from build123d import *

# Parameters (mm, degrees)
BOSS_EXTRUDE1_DEPTH = 38.1
CUT_EXTRUDE1_DEPTH  = 2.54
CUT_EXTRUDE2_DEPTH  = 34.29
BOSS_EXTRUDE2_DEPTH = 25.4
SHELL1_START        = -12.546191045
SHELL1_DEPTH        = 24.13
SHELL1_2_DEPTH      = 22.86


# Read off the part's stored shape, not the designer's step: Shell1
with BuildPart() as part:
    # Sketch1 → Boss-Extrude1 (new body)
    with BuildSketch(Plane(origin=(0, 0, 0), x_dir=(1, 0, 0), z_dir=(0, 1, 0))):
        Polygon((12.853808955, 0.174987325), (12.853808955, 37.417012675), (82.296, 25.146), (82.296, 12.446), align=None)
    extrude(amount=BOSS_EXTRUDE1_DEPTH)

    # Sketch3 → Cut-Extrude1 (cut)
    with BuildSketch(Plane(origin=(0, 35.56, 0), x_dir=(1, 0, 0), z_dir=(0, 1, 0))):
        Polygon((79.756, 14.576512841), (79.756, 23.015487159), (15.393808955, 34.388821586), (15.393808955, 3.203178414), align=None)
    extrude(amount=CUT_EXTRUDE1_DEPTH, mode=Mode.SUBTRACT)

    # Sketch6 → Cut-Extrude2 (cut)
    with BuildSketch(Plane(origin=(0, 35.56, 0), x_dir=(1, 0, 0), z_dir=(0, 1, 0))):
        Polygon((81.026, 13.511256421), (81.026, 24.080743579), (14.123808955, 35.90291713), (14.123808955, 1.68908287), align=None)
    extrude(amount=-CUT_EXTRUDE2_DEPTH, mode=Mode.SUBTRACT)

    # Sketch8 → Boss-Extrude2 (add)
    with BuildSketch(Plane.ZY.offset(-12.853808955)):
        Polygon((-31.26502256, 38.1), (-31.26502256, 0), (-18.796, 2.1986251), (-6.32697744, 0), (-6.32697744, 38.1), (-18.796, 40.2986251), align=None)
    extrude(amount=BOSS_EXTRUDE2_DEPTH)

    # Shell1 outline → Shell1 (cut)
    with BuildSketch(Plane.YZ.offset(SHELL1_START)):
        Polygon((35.56, -28.72502256), (35.56, -8.86697744), (3.027054125, -8.86697744), (4.777808695, -18.796), (3.027054125, -28.72502256), align=None)
    extrude(amount=SHELL1_DEPTH, mode=Mode.SUBTRACT)

    # Shell1 2 outline → Shell1 2 (cut)
    with BuildSketch(Plane.YZ.offset(SHELL1_START)):
        Polygon((35.968686937, -8.86697744), (35.56, -8.86697744), (35.56, -28.72502256), (35.968686937, -28.72502256), (37.719441506, -18.796), align=None)
    extrude(amount=SHELL1_2_DEPTH, mode=Mode.SUBTRACT)


solid = part.part
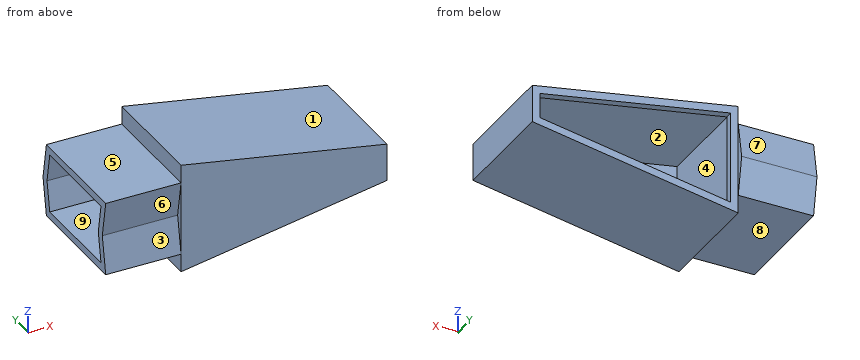
Source: CAD feature listing. Evaluate the final solid. Frame: model axes, mm. Face numbers are marked on the shaded views. A direction names the side the tool comes from. Round coordinates to 2 decimals unless told otherwise and drop trailing zeros. Loops run counter-clockwise (first coordinate to the right, second up) from the corner with the lowest first, then second, coordinate; pieces in that order, holes last. Notation, with made-up numbers: (-22, 29) -> (3, 29) arc R22 ccw to (3, 53) -> close; hole circle Ø5 at (53.5, -28.5). An arc over 180 degrees is marked (long way). Answer as a JSON object with one key per item and string values. Group by question number.
Q1. Section query D-D (x = 55.5). Output: boundary loops of the cut face in (y, z), plus the area to 3 significant figures.
Q2. Mould query, pull axis X, two halves, no side actions, for the marked faces 1, 2, 3 and 4. Classes: pulls with the +X half, pulls with the -X half, needs draft (parallel to the pull), parting line crosses it, or undercut.
Q3. Contact query for flat-ended pins moving along their axis: P1, Ø8, axis at x = 0.5, z = -29, coming from the -Y side; P2, Ø12, axis at x = 25.5, y = 16.5, coming from the -Z side; P3, Ø2.5, axis at y = 39.5, z = -19.5, coming from the +X side. Output: stop coordinate, or through.
Q4. Section query A-A (y = 11). Output: boundary loops of the cut face in (x, z), plus the area to 3 significant figures.
Q5. Access query for the marked faces 5, 6, 7, 8 and 9. Directions: +Z, -Z, +X, -X, +Y, -Y. A direction counts if a zero-diameter tool reaches every point of the face in a straight line with its end or side. Return the directions, or none.
Q6. Section query B-B (x = 71.5). Output: boundary loops of the cut face in (y, z), plus the area to 3 significant figures.
Q7. Ray query, line 1 (Z direction, x = -1.5, y = 10); line 2 (X direction, y = 27, z = -22); line 3 (Y direction, x = 33, z = -17). Return the intervals inside material, ascending. Write a range as from..to.
Q8. Section query C-C (z = -21). Output: boundary loops of the cut face in (x, y), plus the area to 3 significant figures.
Completed:
{
 "1": {"outline": "(0, -29.88) -> (38.1, -29.88) -> (38.1, -27.3) -> (35.56, -27.3) -> (35.56, -28.59) -> (1.27, -28.59) -> (1.27, -9) -> (35.56, -9) -> (35.56, -10.29) -> (38.1, -10.29) -> (38.1, -7.71) -> (0, -7.71) -> close", "area": "130 mm²"},
 "2": {"face 1": "pulls with the +X half", "face 2": "undercut", "face 3": "needs draft", "face 4": "undercut"},
 "3": {"P1": "y = 0", "P2": "z = -36.24", "P3": "x = 12.85"},
 "4": {"outline": "(-12.55, -31.27) -> (12.85, -31.27) -> (12.85, -37.42) -> (82.3, -25.15) -> (82.3, -12.45) -> (12.85, -0.17) -> (12.85, -6.33) -> (-12.55, -6.33) -> (-12.55, -8.87) -> (11.58, -8.87) -> (11.58, -28.73) -> (-12.55, -28.73) -> close; hole (14.12, -35.9) -> (81.03, -24.08) -> (81.03, -13.51) -> (14.12, -1.69) -> close", "area": "390 mm²"},
 "5": {"face 5": "+Z, -X, +Y, -Y", "face 6": "-X, -Y", "face 7": "+Z, +X, -X, +Y", "face 8": "-Z, -X, +Y, -Y", "face 9": "-X"},
 "6": {"outline": "(0, -27.05) -> (38.1, -27.05) -> (38.1, -24.47) -> (35.56, -24.47) -> (35.56, -25.76) -> (1.27, -25.76) -> (1.27, -11.83) -> (35.56, -11.83) -> (35.56, -13.12) -> (38.1, -13.12) -> (38.1, -10.54) -> (0, -10.54) -> close", "area": "123 mm²"},
 "7": {"line 1": "-31.27..-28.73, -8.87..-6.33", "line 2": "11.58..14.12, 81.03..82.3", "line 3": "0..1.27"},
 "8": {"outline": "(-12.55, 1.81) -> (12.85, 1.81) -> (12.85, 0) -> (82.3, 0) -> (82.3, 38.1) -> (79.76, 38.1) -> (79.76, 35.56) -> (81.03, 35.56) -> (81.03, 1.27) -> (14.12, 1.27) -> (14.12, 35.56) -> (15.39, 35.56) -> (15.39, 38.1) -> (12.85, 38.1) -> (12.85, 39.91) -> (-12.55, 39.91) -> (-12.55, 37.33) -> (10.31, 37.33) -> (10.31, 35.56) -> (11.58, 35.56) -> (11.58, 4.39) -> (-12.55, 4.39) -> close", "area": "363 mm²"}
}
